```python
from build123d import *

# Parameters (mm, degrees)
F1_DEPTH = 4
F3_DEPTH = 5
F4_R     = 0.25


with BuildPart() as f1:
    # F0 (on Top) → F1 (new body)
    with BuildSketch(Plane.XY):
        with BuildLine():
            ThreePointArc((0, -2), (-2, 0), (0, 2))
            Line((0, 2), (-8, 2))
            Line((-8, 2), (-8, -2))
            Line((-8, -2), (0, -2))
        make_face()
    extrude(amount=F1_DEPTH)

    # F2 (on face) → F3 (cut)
    with BuildSketch(Plane(origin=(-8, 0, 0), x_dir=(0, -1, 0), z_dir=(-1, 0, 0))):
        with BuildLine():
            ThreePointArc((-1.25, 2), (0, 0.75), (1.25, 2))
            ThreePointArc((1.25, 2), (0, 3.25), (-1.25, 2))
        make_face()
        with BuildLine():
            ThreePointArc((-1.25, 2), (0, 3.25), (1.25, 2))
            Line((1.25, 2), (1.25, 4))
            Line((1.25, 4), (-1.25, 4))
            Line((-1.25, 4), (-1.25, 2))
        make_face()
    extrude(amount=-F3_DEPTH, mode=Mode.SUBTRACT)

    # F4
    f4_edges = [f1.edges().sort_by_distance(p)[0] for p in [
        (0, 2, 2),
        (0, -2, 2),
    ]]
    fillet(f4_edges, radius=F4_R)


solid = f1.part
```
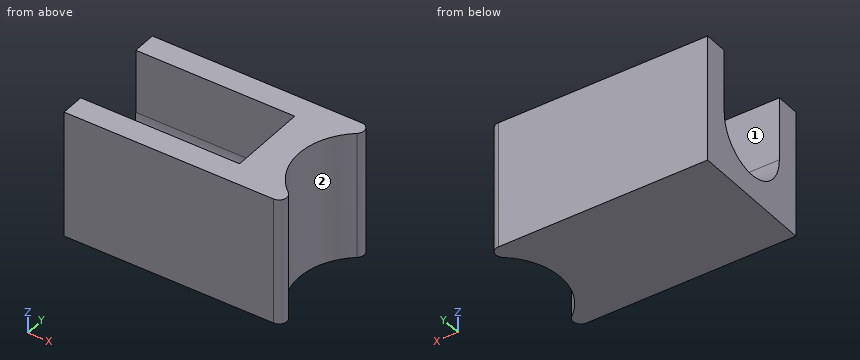
CAD build for the part. Positions are in the model's coordinates, mm. Face numbers are marked on the shaded views. A direction names the side the tool comes from. Round coordinates to 2 decimals unless told otherwise and drop trailing zeros. Order: outer loops, then holes, each group sorted by start corner. A loop starts at its lowest first (then second) coordinate and runs counter-clockwise, first axis right, second up. Notation, with made-up numbers: (69.25, -36) - (109.25, -36) arc R22 ccw to (109.25, -8) - close; hole circle Ø7 at (-18.75, 31). An arc over 180 degrees is marked (long way). Answer as CSV lines item,"result". Start each with the question number.
1. Saw through at C-C, the plane y = -0.7. Write the cut outline in (x, z), and give its area (3 significant figures).
2. Saw through at A-A, the plane x = -6.75. Write the cut outline in (y, z).
3. Drill centre lines: L1, parallel to Y at x = -6, z = 3.75; L2, parallel to Y at x = -3.5, z = 1.25; L3, parallel to X at y = 0.1, z = 0.85. Where is each one in solid material? Low to high. Write a range as [from, to].
4. Saw through at B-B, the plane y = 0. Write the cut outline in (x, z), and give its area (3 significant figures).
5. Pin check, flat tips, straight feed: pin 1 (1 mm diameter, centred on y = -1, z = 2.5, fed in from +X); pin 2 (2 mm diameter, centred on y = 0, z = 3, fed in from -X). Stop position of each tip, or through.
6. Tool access for the marked faces 1 and 2: list every direction of +Z, -Z, +X, -X, +Y, -Y with a clear straight run to the whole face (end or side of a thin tool).
Model answer:
1,outline,"(-8, 0) - (-1.87, 0) - (-1.87, 4) - (-3, 4) - (-3, 0.96) - (-8, 0.96) - close"
1,area,"9.33 mm²"
2,outline,"(-2, 0) - (2, 0) - (2, 4) - (1.25, 4) - (1.25, 2) arc R1.25 cw to (-1.25, 2) - (-1.25, 4) - (-2, 4) - close"
3,L1,"y = [-2, -1.25], [1.25, 2]"
3,L2,"y = [-2, -1], [1, 2]"
3,L3,"x = [-3, -2]"
4,outline,"(-8, 0) - (-2, 0) - (-2, 4) - (-3, 4) - (-3, 0.75) - (-8, 0.75) - close"
4,area,"7.75 mm²"
5,pin 1,"stops at x = -1.32"
5,pin 2,"stops at x = -3"
6,face 1,"+Z, -X"
6,face 2,"+Z, -Z, +X"
